Autodesk Inventor part; units mm, degrees
ref_plane "YZ Plane" through (0, 0, 0) normal (1, 0, 0) x (0, 1, 0)
ref_plane "XZ Plane" through (0, 0, 0) normal (0, 1, 0) x (-1, 0, 0)
ref_plane "XY Plane" through (0, 0, 0) normal (0, 0, 1) x (1, 0, 0)
sketch "Sketch1" plane through (0, 0, 0) normal (0, 1, 0) x (-1, 0, 0)
  line L0 (0, 0) -> (0, -10)
  line L1 (0, -10) -> (10, -10)
  line L2 (10, -10) -> (10, 0)
  line L3 (10, 0) -> (0, 0)
  dimension "d0" = 10
  dimension "d1" = 10
extrude "Extrusion1" add sketch "Sketch1" along normal blind 8
sketch "Sketch2" plane through (0, 8, 0) normal (0, 1, 0) x (1, 0, 0)
  line L0 (-10, 10) -> (-10, 0)
  line L1 (-10, 0) -> (0, 0)
  line L2 (-10, 10) -> (0, 0)
  line L3 (0, 0) -> (-10, 0)
  line L4 (-10, 0) -> (0, 10)
  circle A0 centre (-5, 5) radius 2.6
  dimension "d4" = 5.2
extrude "Extrusion2" cut sketch "Sketch2" against normal through all contours A0 L4 L2 | L2 L4 A0 | L4 L2 A0 | L4 A0 L2
chamfer "Chamfer1" distance 2 distance2 3 1 edges at (-7.6, 0, -5) measured on face at (-5.1045, 0, -9.1937)
sketch "Sketch3" plane through (-10, 0, 0) normal (0, 0, 1) x (1, 0, 0)
  line L0 (7.6, 8) -> (7.6, 3)
  line L1 (7.6, 8) -> (10, 8)
  line L2 (10, 8) -> (10, 0)
  line L3 (10, 0) -> (7.6, 0)
  line L4 (0, 0) -> (10, 0)
  line L5 (2.4, 8) -> (7.6, 8)
  line L6 (7.6, 8) -> (7.6, 0)
  line L7 (0, 8) -> (10, 8)
  line L8 (10, 0) -> (10, 8)
  line L9 (0, 8) -> (10, 0)
  line L10 (10, 0) -> (0, 0)
  line L11 (10, 8) -> (0, 0)
  circle A0 centre (5, 4) radius 1.1
  dimension "d10" = 2.2
extrude "Extrusion3" cut sketch "Sketch3" against normal through all contours A0 L9 L11 | L11 L9 A0 | L11 A0 L9 | L9 A0 L11
fillet "Fillet1" radius 2.5 2 edges at (0, 0, -5) (-10, 0, -5)
sketch "Sketch4" plane through (0, 8, 0) normal (0, 1, 0) x (1, 0, 0)
  arc A0 (-4.5417, 2.4407) -> (-4.5417, 7.5593) centre (-5, 5) ccw
  line L0 (-5, 5) -> (0, 5)
  line L1 (0, 0) -> (0, 10)
  line L2 (0, 5) -> (0, 8)
  line L3 (0, 8) -> (-10, 8)
  line L4 (-10, 10) -> (-10, 0)
  line L5 (-10, 8) -> (-10, 0)
  line L6 (-10, 0) -> (0, 0)
  line L7 (0, 0) -> (0, 8)
  line L8 (0, 10) -> (-10, 10)
  line L9 (0, 8) -> (0, 10)
  line L10 (0, 10) -> (-10, 10)
  line L11 (-10, 10) -> (-10, 8)
  line L12 (-10, 0) -> (-10, 0)
  line L13 (0, 0) -> (-2.5, 0)
  line L14 (-10, 0) -> (0, 0)
  line L15 (0, 0) -> (0, 0)
  line L16 (-10, 0) -> (-10, 10)
  line L17 (-10, 5) -> (-10, 9)
  line L18 (-10, 9) -> (-10, 1)
  line L19 (-10, 1) -> (0, 1)
  line L20 (0, 10) -> (0, 0)
  line L21 (-10, 9) -> (0, 9)
  point P0 (0, 0)
  point P1 (-10, 0)
  dimension "d14" = 3
  dimension "d15" = 8
  dimension "d18" = 8
extrude "Extrusion4" cut sketch "Sketch4" against normal through all contours L6 L4 L19 L1 | L21 L4 L8 L1
properties part number "pist-dolni"
Work out the finished part from the listing and answer in its coordinate system (mm). Give positions to 0.01 mm unless a question says otherwise; leave off trailing zeros. Write each loop counter-clockwise with the first axis right and the second up, starting at its lowest first coordinate (ties: lowest second). Pieces come first, ordered by that corner, then holes.
(1) The mould has two halves that part along Y. Classify faces 1 (the cylindrical face through (-4.41, 4.93, -8.17)), 2 (the flat face through (-5, 8, -2)), 3 (the flat face through (-6, 5, -1)), 4 (the cylindrical face through (-4.492, 3.024, -1.811)): pulls with the +Y half, pulls with the -Y half, needs draft (parallel to the pull), parting line crosses it, or undercut.
Final values:
face 1: undercut
face 2: pulls with the +Y half
face 3: needs draft
face 4: undercut
(2) The part is cut by section B-B on x = -5. Write down the section's boundary in (y, z).
Final values:
outline: (0.9, -9) - (2.9, -9) - (2.9, -7.67) - close; (0.9, -1) - (2.9, -2.33) - (2.9, -1) - close; (5.1, -9) - (8, -9) - (8, -7.6) - (5.1, -7.6) - close; (5.1, -2.4) - (8, -2.4) - (8, -1) - (5.1, -1) - close
(3) The part is cut by section A-A on y = 4. Write down the section's boundary in (x, z), plus the area to 3 significant figures.
Final values:
outline: (-10, -9) - (-6.1, -9) - (-6.1, -7.36) arc R2.6 cw to (-6.1, -2.64) - (-6.1, -1) - (-10, -1) - close; (-3.9, -9) - (0, -9) - (0, -1) - (-3.9, -1) - (-3.9, -2.64) arc R2.6 cw to (-3.9, -7.36) - close
area: 52.3 mm2
(4) The part is cut by section D-D on z = -5. Write down the section's boundary in (x, y).
Final values:
outline: (-10, 2.5) arc R2.5 ccw to (-9.17, 0.64) - (-7.6, 3) - (-7.6, 8) - (-10, 8) - close; (-2.4, 3) - (-0.83, 0.64) arc R2.5 ccw to (0, 2.5) - (0, 8) - (-2.4, 8) - close
(5) Straight lines are drawn through the part: line 1 (X direction, y = 4, z = -8.05); line 2 (Z direction, x = -6.5, y = 4); line 3 (Z direction, x = -2.75, y = 1.5). For each, find the intervals that lie inside material, in ascending order.
Final values:
line 1: x = -10 to -6.1, -3.9 to 0
line 2: z = -9 to -7.12, -2.88 to -1
line 3: z = -9 to -7.81, -2.19 to -1
(6) The part is cut by section C-C on y = 6.75. Write down the section's boundary in (x, z), plus the area to 3 significant figures.
Final values:
outline: (-10, -9) - (0, -9) - (0, -1) - (-10, -1) - close; hole circle Ø5.2 at (-5, -5)
area: 58.8 mm2
(7) Flat-ended cylindrical pins translate along their axes: pin 1 Ø4 at (x, z) = (-4.5, -4) entering from -Y; pin 2 Ø3 at (x, z) = (-9, -7.5) entering from -Y; pin 3 Ø4.5 at (x, z) = (-5, -5) entering from +Y. Find the tip coordinate at first contact, or state that the pin passes through.
Final values:
pin 1: stops at y = 2.22
pin 2: stops at y = 0.03
pin 3: passes through
